Here's the drawing with two shaded views (mm, measured from the low corner). I have some questions. Round coordinates to 2 decimals unless told otherwise and drop trailing zeros. Write each loop counter-clockwise with the first axis right and the second up, starting at its lowest first coordinate (ties: lowest second). Pieces come first, ordered by that corner, then holes. Notation, with made-up numbers: (16, 63.5) -> (71, 63.5) arc R19 ccw to (71, 77.5) -> close; hole circle Ø1 at (81.5, 10.25). An arc over 180 degrees is marked (long way). Use CSV: the item, a comma, the result in double quotes.
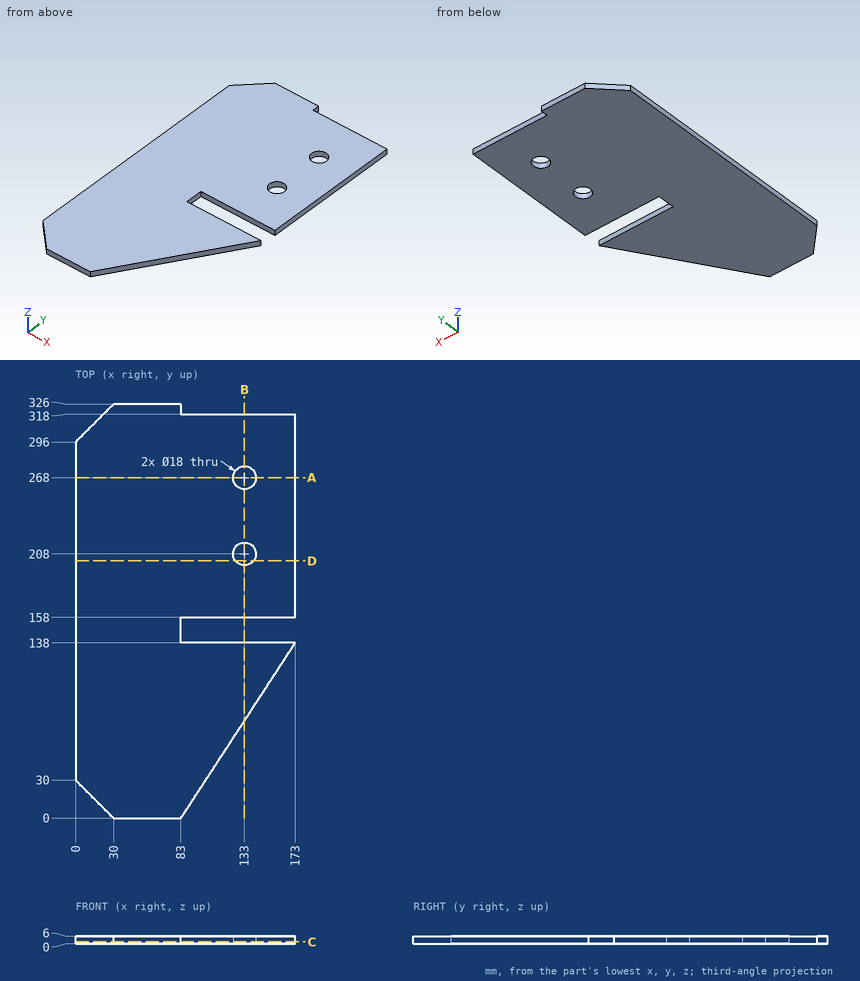
Q1. Suppose I cut it at D-D (y = 202.5). Write out the boundary of the cut face in (x, z), and give its area (3 significant figures).
Resolved:
outline,"(0, 0) -> (125.88, 0) -> (125.88, 6) -> (0, 6) -> close; (140.12, 0) -> (173, 0) -> (173, 6) -> (140.12, 6) -> close"
area,"953 mm^2"
Q2. Please list where these lines run through material, in increasing order: probe 1 along X at (y, z) = (268, 2.3); probe 2 along X at (y, z) = (141, 0.9); probe 3 along Y at (x, z) = (133, 1.45).
Resolved:
probe 1,"x = 0 to 124, 142 to 173"
probe 2,"x = 0 to 83"
probe 3,"y = 76.67 to 138, 158 to 199, 217 to 259, 277 to 318"
Q3. Suppose I cut it at A-A (y = 268). Write out the boundary of the cut face in (x, z).
Resolved:
outline,"(0, 0) -> (124, 0) -> (124, 6) -> (0, 6) -> close; (142, 0) -> (173, 0) -> (173, 6) -> (142, 6) -> close"
Q4. Suppose I cut it at C-C (z = 1.6). Write out the boundary of the cut face in (x, y).
Resolved:
outline,"(0, 30) -> (30, 0) -> (83, 0) -> (173, 138) -> (83, 138) -> (83, 158) -> (173, 158) -> (173, 318) -> (83, 318) -> (83, 326) -> (30, 326) -> (0, 296) -> close; hole circle Ø18 at (133, 208); hole circle Ø18 at (133, 268)"
Q5. Suppose I cut it at B-B (x = 133). Write out the boundary of the cut face in (y, z), and give its area (3 significant figures).
Resolved:
outline,"(76.67, 0) -> (138, 0) -> (138, 6) -> (76.67, 6) -> close; (158, 0) -> (199, 0) -> (199, 6) -> (158, 6) -> close; (217, 0) -> (259, 0) -> (259, 6) -> (217, 6) -> close; (277, 0) -> (318, 0) -> (318, 6) -> (277, 6) -> close"
area,"1,110 mm^2"
Q6. Will these pins go through, and if not, where does the flat tip stop? P1, Ø2, axis at x = 111, z = 3, coming from the +Y side; P2, Ø16, axis at x = 133, y = 268, coming from the +Z side.
Resolved:
P1,"stops at y = 318"
P2,"passes through"
